Geometry check sheet. Reference: the model listing, model coordinates, mm. Face numbers are marked on the shaded views. A direction names the side the tool comes from. Round coordinates to 2 decimals unless told otherwise and drop trailing zeros. Write each loop counter-clockwise with the first axis right and the second up, starting at its lowest first coordinate (ties: lowest second). Pieces come first, ordered by that corner, then holes. Notation, with made-up numbers: (-8, 46.5) - (28, 46.5) arc R16 cw to (28, 72.5) - close; hole circle Ø11 at (25, 13.5). An arc over 180 degrees is marked (long way). Return JSON: item names as keys, results as strings. Group by question number.
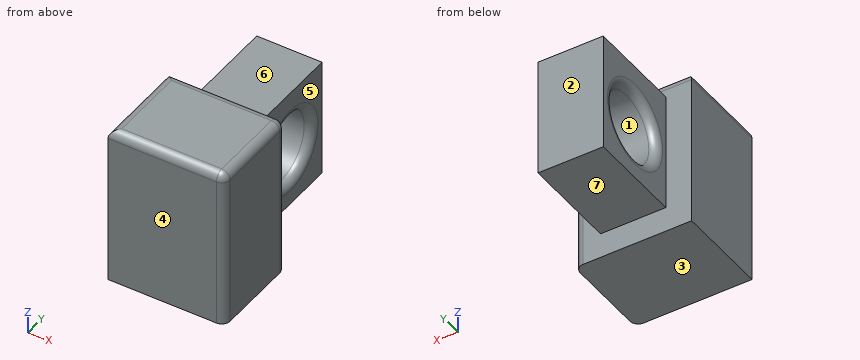
from build123d import *

# Parameters (mm, degrees)
F0_W     = 70.792555
F0_H     = 56.937516
F1_DEPTH = 97.26762
F2_R     = 5.08
F3_R     = 5.08
F4_W     = 39.581746
F4_H     = 72.326273
F5_DEPTH = 58.996573
F6_R     = 20.976362
F7_DEPTH = 77.683359
F8_R     = 5.08


with BuildPart() as f1:
    # F0 (on Top) → F1 (new body)
    with BuildSketch(Plane.XY):
        with Locations((51.602363, 28.468758)):
            Rectangle(F0_W, F0_H)
    extrude(amount=F1_DEPTH)

    # F2
    f2_edges = [f1.edges().sort_by_distance(p)[0] for p in [
        (86.998641, 28.468758, 97.26762),
    ]]
    fillet(f2_edges, radius=F2_R)

    # F3
    f3_edges = [f1.edges().sort_by_distance(p)[0] for p in [
        (16.206086, 28.468758, 97.26762),
        (49.062364, 0, 97.26762),
        (49.062364, 56.937516, 97.26762),
    ]]
    fillet(f3_edges, radius=F3_R)

    # F4 (on face) → F5 (join)
    with BuildSketch(Plane(origin=(0, 56.937516, 0), x_dir=(-1, 0, 0), z_dir=(0, 1, 0))):
        with Locations((-51.677324, 51.547486)):
            Rectangle(F4_W, F4_H)
    extrude(amount=F5_DEPTH)

    # F6 (on face) → F7 (cut)
    with BuildSketch(Plane(origin=(31.886451, 0, 0), x_dir=(0, -1, 0), z_dir=(-1, 0, 0))):
        with Locations((-86.047255, 50.220259)):
            Circle(F6_R)
    extrude(amount=-F7_DEPTH, mode=Mode.SUBTRACT)

    # F8
    f8_edges = [f1.edges().sort_by_distance(p)[0] for p in [
        (71.468197, 107.023617, 50.220259),
        (31.886451, 107.023617, 50.220259),
    ]]
    fillet(f8_edges, radius=F8_R)


solid = f1.part
1. Section check B-B (x = 64.5). Enter the section's corners in (y, z), and give its area (3 significant figures).
2. Section check A-A (x = 27.5). Enter the section's corners in (y, z).
3. Material ranges on line 1 along Y through (x, z) = (60.5, 4); line 2 along X through (y, z) = (78, 21.5); line 3 along Z through (x, y) = (64, 100), recorded low to high.
4. Tool access check on the marked faces 5, 6 and 7. Record the directions out of +Z, -Z, +X, -X, +Y, -Y that give a thin tool (end or side, any length) a straight path to the whole face; none if there is none.
5. Depth check by flat-ended pin: pin 1 Ø5 at (y, z) = (62.5, 21) entering from +X; pin 2 Ø12 at (x, y) = (50, 87.5) entering from -Z; pin 3 Ø1.5 at (x, y) = (40, 27) entering from -Z; pin 4 Ø1.5 at (y, z) = (58.5, 58) entering from -X. Enter the tip coordinate at first touch or a pass-through.
6. Mould release check, pull along Y, two halves, no side actions. Record for the marked faces 1, 2, 3 and 4: pulls with the +Y half, pulls with the -Y half, needs draft (parallel to the pull), parting line crosses it, or undercut.
Result sheet:
{
 "1": {"outline": "(0, 0) - (56.94, 0) - (56.94, 15.38) - (115.93, 15.38) - (115.93, 87.71) - (56.94, 87.71) - (56.94, 92.19) arc R5.08 ccw to (51.86, 97.27) - (5.08, 97.27) arc R5.08 ccw to (0, 92.19) - close; hole circle Ø41.95 at (86.05, 50.22)", "area": "8,410 mm²"},
 "2": {"outline": "(0, 0) - (56.94, 0) - (56.94, 92.19) arc R5.08 ccw to (51.86, 97.27) - (5.08, 97.27) arc R5.08 ccw to (0, 92.19) - close"},
 "3": {"line 1": "y = 0 to 56.94", "line 2": "x = 31.89 to 71.47", "line 3": "z = 15.38 to 34.56, 65.88 to 87.71"},
 "4": {"face 5": "+Z, -Z, +X, +Y", "face 6": "+Z, +X, -X, +Y", "face 7": "-Z, +X, -X, +Y"},
 "5": {"pin 1": "stops at x = 71.47", "pin 2": "stops at z = 15.38", "pin 3": "stops at z = 0", "pin 4": "stops at x = 31.89"},
 "6": {"face 1": "undercut", "face 2": "pulls with the +Y half", "face 3": "needs draft", "face 4": "pulls with the -Y half"}
}
